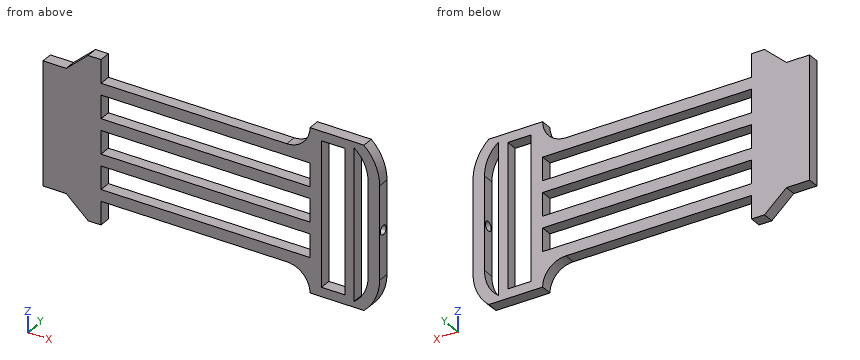
```python
from build123d import *

# Parameters (mm, degrees)
Y_KSEKLIK_EKSTR_ZYON1_DEPTH = 7
IZIM2_R                     = 1.5
KES_EKSTR_ZYON1_DEPTH       = 7
PAH1_SIZE                   = 2.5
IZIM3_R                     = 2
KES_EKSTR_ZYON2_DEPTH       = 10
KES_EKSTR_ZYON3_START       = -10
IZIM4_R                     = 2
KES_EKSTR_ZYON3_DEPTH       = 10
RADYUS1_R                   = 20
IZIM5_W                     = 90
IZIM5_H                     = 10
IZIM5_W_2                   = 10
IZIM5_H_2                   = 70
KES_EKSTR_ZYON4_DEPTH       = 10
RADYUS2_R                   = 4
KES_EKSTR_ZYON5_DEPTH       = 10
IZIM8_W                     = 5
IZIM8_H                     = 53
KES_EKSTR_ZYON6_DEPTH       = 10
IZIM9_W                     = 8.724341423
IZIM9_H                     = 2.178581573
IZIM9_W_2                   = 9.164333206
Y_KSEKLIK_EKSTR_ZYON2_DEPTH = 10
IZIM10_W                    = 140
IZIM10_H                    = 10
KES_EKSTR_ZYON7_DEPTH       = 10
IZIM11_W                    = 10
IZIM11_H                    = 4
Y_KSEKLIK_EKSTR_ZYON3_DEPTH = 7
RADYUS3_R                   = 10
IZIM12_W                    = 4
IZIM12_H                    = 7
Y_KSEKLIK_EKSTR_ZYON4_DEPTH = 7
RADYUS4_R                   = 5
IZIM13_R                    = 1.5
KES_EKSTR_ZYON8_DEPTH       = 7
PAH2_SIZE                   = 1.5
RADYUS5_R                   = 2
IZIM14_W                    = 144.535934645
IZIM14_H                    = 70
KES_EKSTR_ZYON9_DEPTH       = 2
RADYUS6_R                   = 2
IZIM16_R                    = 2
KES_EKSTR_ZYON11_DEPTH      = 7
KES_EKSTR_ZYON12_DEPTH      = 10


# Some blends are built 0.0001 mm under size
with BuildPart() as part:
    # izim1 → Y_kseklik-Ekstr_zyon1 (new body)
    with BuildSketch(Plane(origin=(0, 0, 0), x_dir=(1, 0, 0), z_dir=(0, 1, 0))):
        Polygon((0, 0), (0, 53), (15, 53), (30, 66.5), (150, 66.5), (150, -13.5), (30, -13.5), (15, 0), align=None)
    extrude(amount=Y_KSEKLIK_EKSTR_ZYON1_DEPTH)

    # izim2 → Kes-Ekstr_zyon1 (cut)
    with BuildSketch(Plane(origin=(0, 7, 0), x_dir=(1, 0, 0), z_dir=(0, 1, 0))):
        with Locations(Location((2.5, 41.25, 0), (0, 0, 270))):
            Circle(IZIM2_R)
        with Locations(Location((2.5, 11.75, 0), (0, 0, 270))):
            Circle(IZIM2_R)
    extrude(amount=-KES_EKSTR_ZYON1_DEPTH, mode=Mode.SUBTRACT)

    # Pah1
    # the kernel refuses this chamfer: 2.5 mm, written as the material it takes off along each edge
    with BuildSketch(Plane(origin=(2.5, 7, -41.25), x_dir=(0, 0, 1), z_dir=(-1, 0, 0))) as pah1_piece_1:
        Polygon((1.5 + PAH1_SIZE, 0), (1.5, -PAH1_SIZE), (1.5, 0), align=None)
    revolve(axis=Axis((2.5, 7, -41.25), (0, 1, 0)), mode=Mode.SUBTRACT)
    with BuildSketch(Plane(origin=(2.5, 7, -11.75), x_dir=(0, 0, 1), z_dir=(-1, 0, 0))) as pah1_piece_2:
        Polygon((1.5 + PAH1_SIZE, 0), (1.5, -PAH1_SIZE), (1.5, 0), align=None)
    revolve(axis=Axis((2.5, 7, -11.75), (0, 1, 0)), mode=Mode.SUBTRACT)

    # izim3 → Kes-Ekstr_zyon2 (cut)
    with BuildSketch(Plane.XY.offset(13.5)):
        with Locations((46.24, 3.5)):
            Circle(IZIM3_R)
    extrude(amount=-KES_EKSTR_ZYON2_DEPTH, mode=Mode.SUBTRACT)

    # izim4 → Kes-Ekstr_zyon3 (cut)
    with BuildSketch(Plane(origin=(0, 0, -66.5), x_dir=(-1, 0, 0), z_dir=(0, 0, -1)).offset(KES_EKSTR_ZYON3_START)):
        with Locations(Location((-46.24, 3.5, 0), (0, 0, 180))):
            Circle(IZIM4_R)
    extrude(amount=KES_EKSTR_ZYON3_DEPTH, mode=Mode.SUBTRACT)

    # Radyus1
    radyus1_edges = [part.edges().sort_by_distance(p)[0] for p in [
        (150, 3.5, -66.5),
        (150, 3.5, 13.5),
    ]]
    fillet(radyus1_edges, radius=RADYUS1_R)

    # izim5 → Kes-Ekstr_zyon4 (cut)
    with BuildSketch(Plane(origin=(0, 7, 0), x_dir=(1, 0, 0), z_dir=(0, 1, 0))):
        with Locations((75, -3.5)):
            Rectangle(IZIM5_W, IZIM5_H)
        with Locations((75, 26.5)):
            Rectangle(IZIM5_W, IZIM5_H)
        with Locations((75, 41.5)):
            Rectangle(IZIM5_W, IZIM5_H)
        with Locations((75, 56.5)):
            Rectangle(IZIM5_W, IZIM5_H)
        with Locations((75, 11.5)):
            Rectangle(IZIM5_W, IZIM5_H)
        with Locations((130, 26.5)):
            Rectangle(IZIM5_W_2, IZIM5_H_2)
    extrude(amount=-KES_EKSTR_ZYON4_DEPTH, mode=Mode.SUBTRACT)

    # Radyus2
    radyus2_edges = [part.edges().sort_by_distance(p)[0] for p in [
        (135, 3.5, -61.5),
        (135, 3.5, 8.5),
    ]]
    fillet(radyus2_edges, radius=RADYUS2_R)

    # izim6 → Kes-Ekstr_zyon5 (cut)
    with BuildSketch(Plane(origin=(0, 7, 0), x_dir=(1, 0, 0), z_dir=(0, 1, 0))):
        with BuildLine():
            Line((139, -6), (139, 59))
            ThreePointArc((139, 59), (143.530979443, 53.484870133), (145, 46.5))
            Line((145, 46.5), (145, 6.5))
            ThreePointArc((145, 6.5), (143.530979443, -0.484870133), (139, -6))
        make_face()
    extrude(amount=-KES_EKSTR_ZYON5_DEPTH, mode=Mode.SUBTRACT)

    # izim8 → Kes-Ekstr_zyon6 (cut)
    with BuildSketch(Plane(origin=(0, 7, 0), x_dir=(1, 0, 0), z_dir=(0, 1, 0))):
        with Locations((2.5, 26.5)):
            Rectangle(IZIM8_W, IZIM8_H)
    extrude(amount=-KES_EKSTR_ZYON6_DEPTH, mode=Mode.SUBTRACT)

    # izim9 → Y_kseklik-Ekstr_zyon2 (add)
    with BuildSketch(Plane.ZY.offset(-5)):
        with Locations((-12.430411948, 5.910709214)):
            Rectangle(IZIM9_W, IZIM9_H)
        with Locations((-41.247168871, 5.910709214)):
            Rectangle(IZIM9_W_2, IZIM9_H)
    extrude(amount=-Y_KSEKLIK_EKSTR_ZYON2_DEPTH)

    # izim10 → Kes-Ekstr_zyon7 (cut)
    with BuildSketch(Plane(origin=(0, 7, 0), x_dir=(1, 0, 0), z_dir=(0, 1, 0))):
        with Locations((85, -13.5)):
            Rectangle(IZIM10_W, IZIM10_H)
        with Locations((85, 66.5)):
            Rectangle(IZIM10_W, IZIM10_H)
    extrude(amount=-KES_EKSTR_ZYON7_DEPTH, mode=Mode.SUBTRACT)


with BuildPart() as kes_ekstr_zyon7_piece_1:
    # of the separate pieces the step leaves, piece 1, a body of its own (kes_ekstr_zyon7_pieces)
    add(part.part.solids().sort_by_distance((24.444444444, 0, 8.5))[0])



with BuildPart() as kes_ekstr_zyon7_piece_2:
    # of the separate pieces the step leaves, piece 2, a body of its own (kes_ekstr_zyon7_pieces)
    add(part.part.solids().sort_by_distance((143.228756555, 0, 8.5))[0])


with BuildPart() as kes_ekstr_zyon7_piece_1_1:
    add(kes_ekstr_zyon7_piece_1.part)

    add(kes_ekstr_zyon7_piece_2.part)  # Y_kseklik-Ekstr_zyon3 merges Kes-Ekstr_zyon7 piece 2
    # izim11 → Y_kseklik-Ekstr_zyon3 (add)
    with BuildSketch(Plane(origin=(0, 7, 0), x_dir=(1, 0, 0), z_dir=(0, 1, 0))):
        with Locations((130, -6.5)):
            Rectangle(IZIM11_W, IZIM11_H)
        with Locations((130, 59.5)):
            Rectangle(IZIM11_W, IZIM11_H)
    extrude(amount=-Y_KSEKLIK_EKSTR_ZYON3_DEPTH)

    # Radyus3
    radyus3_edges = [kes_ekstr_zyon7_piece_1_1.edges().sort_by_distance(p)[0] for p in [
        (120, 3.5, -1.5),
        (120, 3.5, -51.5),
    ]]
    fillet(radyus3_edges, radius=RADYUS3_R - 0.0001)  # a hair under: the kernel refuses the full size

    # izim12 → Y_kseklik-Ekstr_zyon4 (add)
    with BuildSketch(Plane(origin=(0, 7, 0), x_dir=(1, 0, 0), z_dir=(0, 1, 0))):
        with Locations((7, 15)):
            Rectangle(IZIM12_W, IZIM12_H)
        with Locations((7, 38)):
            Rectangle(IZIM12_W, IZIM12_H)
    extrude(amount=Y_KSEKLIK_EKSTR_ZYON4_DEPTH)

    # Radyus4
    radyus4_edges = [kes_ekstr_zyon7_piece_1_1.edges().sort_by_distance(p)[0] for p in [
        (7, 7, -11.5),
        (7, 7, -18.5),
        (7, 7, -34.5),
        (7, 7, -41.5),
    ]]
    fillet(radyus4_edges, radius=RADYUS4_R)

    # izim13 → Kes-Ekstr_zyon8 (cut)
    with BuildSketch(Plane.ZY.offset(-5)):
        with Locations((-38, 10.5)):
            Circle(IZIM13_R)
        with Locations((-15, 10.5)):
            Circle(IZIM13_R)
    extrude(amount=-KES_EKSTR_ZYON8_DEPTH, mode=Mode.SUBTRACT)

    # Pah2
    pah2_edges = [kes_ekstr_zyon7_piece_1_1.edges().sort_by_distance(p)[0] for p in [
        (9, 10.5, -39.5),
        (9, 10.5, -16.5),
    ]]
    chamfer(pah2_edges, length=PAH2_SIZE)

    # Radyus5
    radyus5_edges = [kes_ekstr_zyon7_piece_1_1.edges().sort_by_distance(p)[0] for p in [
        (7, 14, -41.5),
        (7, 14, -34.5),
        (7, 14, -11.5),
        (7, 14, -18.5),
    ]]
    fillet(radyus5_edges, radius=RADYUS5_R - 0.0001)  # a hair under: the kernel refuses the full size

    # izim14 → Kes-Ekstr_zyon9 (cut)
    with BuildSketch(Plane(origin=(0, 7, 0), x_dir=(1, 0, 0), z_dir=(0, 1, 0))):
        with Locations((81.267967322, 26.5)):
            Rectangle(IZIM14_W, IZIM14_H)
    extrude(amount=-KES_EKSTR_ZYON9_DEPTH, mode=Mode.SUBTRACT)

    # Radyus6
    radyus6_edges = [kes_ekstr_zyon7_piece_1_1.edges().sort_by_distance(p)[0] for p in [
        (7, 7, -53),
        (7, 7, 0),
    ]]
    fillet(radyus6_edges, radius=RADYUS6_R)

    # izim16 → Kes-Ekstr_zyon11 (cut)
    with BuildSketch(Plane(origin=(150, 0, 0), x_dir=(0, 0, -1), z_dir=(1, 0, 0))):
        with Locations((26.5, 2.5)):
            Circle(IZIM16_R)
    extrude(amount=-KES_EKSTR_ZYON11_DEPTH, mode=Mode.SUBTRACT)

    # izim17 → Kes-Ekstr_zyon12 (cut)
    with BuildSketch(Plane(origin=(9, 0, 0), x_dir=(0, 0, -1), z_dir=(1, 0, 0))):
        with BuildLine():
            Line((0, 5), (53, 5))
            ThreePointArc((53, 5), (52.414213562, 6.414213562), (51, 7))
            Line((51, 7), (46.5, 7))
            ThreePointArc((46.5, 7), (42.964466094, 8.464466094), (41.5, 12))
            ThreePointArc((41.5, 12), (40.914213562, 13.414213562), (39.5, 14))
            Line((39.5, 14), (36.5, 14))
            ThreePointArc((36.5, 14), (35.085786438, 13.414213562), (34.5, 12))
            ThreePointArc((34.5, 12), (33.035533906, 8.464466094), (29.5, 7))
            Line((29.5, 7), (23.5, 7))
            ThreePointArc((23.5, 7), (19.964466094, 8.464466094), (18.5, 12))
            ThreePointArc((18.5, 12), (17.914213562, 13.414213562), (16.5, 14))
            Line((16.5, 14), (13.5, 14))
            ThreePointArc((13.5, 14), (12.085786438, 13.414213562), (11.5, 12))
            ThreePointArc((11.5, 12), (10.035533906, 8.464466094), (6.5, 7))
            Line((6.5, 7), (2, 7))
            ThreePointArc((2, 7), (0.585786438, 6.414213562), (0, 5))
        make_face()
    extrude(amount=-KES_EKSTR_ZYON12_DEPTH, mode=Mode.SUBTRACT)


with BuildPart() as kes_ekstr_zyon12_kept_piece:
    # of the separate pieces the step leaves, the one the design keeps (kes_ekstr_zyon12_pieces_kept)
    add(kes_ekstr_zyon7_piece_1_1.part.solids().sort_by_distance((5, 5, 0))[0])


solid = kes_ekstr_zyon12_kept_piece.part
```
Check sheet for the modelled part. Datum: model origin and axes. Units: mm. Round coordinates to 2 decimals unless told otherwise and drop trailing zeros. Loops run counter-clockwise (first coordinate to the right, second up) from the corner with the lowest first, then second, coordinate; pieces in that order, holes last. Notation, with made-up numbers: M 78,66 L 113,66 A14 ccw 113,90 Z; hole C 55,80.5 d3. An arc over 180 degrees is marked long. Answer as a JSON object with one key per item and string values.
1. Section check D-D (y = 2.5). State how many separate pieces and enclosed holes the cut face has, plus the area to 3 significant figures.
Reply:
{"separate pieces": "1", "enclosed holes": "4", "area": "4,390 mm²"}
2. Scan lines: line 1 (X direction, y = 2.35, z = -35); line 2 (Z direction, x = 100, y = 2.35); line 3 (X direction, y = 4.2, z = -12). Record each from-to range of solid material in increasing order.
Reply:
{"line 1": "x = 5 to 125, 135 to 139, 145 to 150", "line 2": "z = -51.5 to -46.5, -36.5 to -31.5, -21.5 to -16.5, -6.5 to -1.5", "line 3": "x = 5 to 30, 120 to 125, 135 to 139, 145 to 150"}
3. Section check A-A (z = -26.5). Record the boundary of the cut face in (x, y), plus the area to 3 significant figures.
Reply:
{"outline": "M 5,0 L 30,0 L 30,5 L 5,5 Z; M 120,0 L 125,0 L 125,5 L 120,5 Z; M 135,0 L 139,0 L 139,5 L 135,5 Z; M 145,0 L 150,0 L 150,0.5 L 145,0.5 Z; M 145,4.5 L 150,4.5 L 150,5 L 145,5 Z", "area": "175 mm²"}
4. Section check C-C (x = 113.5). Record the boundary of the cut face in (y, z).
Reply:
{"outline": "M 0,-52.13 L 5,-52.13 L 5,-46.5 L 0,-46.5 Z; M 0,-36.5 L 5,-36.5 L 5,-31.5 L 0,-31.5 Z; M 0,-21.5 L 5,-21.5 L 5,-16.5 L 0,-16.5 Z; M 0,-6.5 L 5,-6.5 L 5,-0.87 L 0,-0.87 Z"}
5. Gauge pin test, flat ends, axial feed: P1, Ø1.5, axis at x = 79.5, z = -44, coming from the -Y side; P2, Ø2.5, axis at x = 91.5, y = 2.5, coming from the +Z side; P3, Ø1.5, axis at x = 82.5, y = 3.5, coming from the -Z side; P4, Ø3, axis at y = 2.5, z = -26.5, coming from the +X side. Record the tip position at first contact, or that the pin passes through.
Reply:
{"P1": "passes through", "P2": "stops at z = -1.5", "P3": "stops at z = -51.5", "P4": "stops at x = 139"}
6. Section check B-B (z = -18.5). Record the boundary of the cut face in (x, y), plus the area to 3 significant figures.
Reply:
{"outline": "M 5,0 L 125,0 L 125,5 L 5,5 Z; M 135,0 L 139,0 L 139,5 L 135,5 Z; M 145,0 L 150,0 L 150,5 L 145,5 Z", "area": "645 mm²"}
